from build123d import *

# Parameters (mm, degrees)
F1_DEPTH = 60
F2_W     = 3
F2_H     = 3
F3_DEPTH = 60
F4_DEPTH = 42
F5_DEPTH = 35
F6_DEPTH = 7


with BuildPart() as f1:
    # F0 (on Front) → F1 (new body)
    with BuildSketch(Plane.XZ):
        with BuildLine():
            Line((-6, 0), (0, 0))
            Line((0, 0), (0, 3))
            Line((0, 3), (-6.3828637444, 3.5))
            ThreePointArc((-6.3828637444, 3.5), (-7.5200895217, 3.1043228005), (-8, 2))
            ThreePointArc((-8, 2), (-7.4142135624, 0.5857864376), (-6, 0))
        make_face()
    extrude(amount=F1_DEPTH)

    # F2 (on face) → F3 (join)
    with BuildSketch(Plane.XZ.offset(60)):
        with Locations((1.5, 1.5)):
            Rectangle(F2_W, F2_H)
    extrude(amount=-F3_DEPTH)

    # F4 (cut): a face of the model
    f4_faces = [f1.faces().sort_by_distance(p)[0] for p in [
        (-2.4940313384, -60, 1.6228930979),
    ]]
    extrude(f4_faces, amount=-F4_DEPTH, mode=Mode.SUBTRACT)

    # F5 (add): a face of the model
    f5_faces = [f1.faces().sort_by_distance(p)[0] for p in [
        (-2.4940313384, -18, 1.6228930979),
    ]]
    extrude(f5_faces, amount=F5_DEPTH)

    # F6 (add): a face of the model
    f6_faces = [f1.faces().sort_by_distance(p)[0] for p in [
        (-2.4940313384, -53, 1.6228930979),
    ]]
    extrude(f6_faces, amount=F6_DEPTH)


solid = f1.part
For this review, take the finished solid that the model builds, in its own axes (mm). A direction names the side the tool comes from. Round coordinates to 2 decimals unless told otherwise and drop trailing zeros. Write each loop counter-clockwise with the first axis right and the second up, starting at its lowest first coordinate (ties: lowest second). Pieces come first, ordered by that corner, then holes. Notation, with made-up numbers: (72.25, 28.25) -> (123.25, 28.25) arc R13 cw to (123.25, 50.25) -> close; hole circle Ø1 at (75, 54). An arc over 180 degrees is marked (long way). Put each result on its own line as item: value.
Q1. To check wall thickness, follow L1, parallel to Z at x = 1.5, y = -7; L2, parallel to X at y = -21.5, z = 2.2; L3, parallel to Z at x = -7.25, y = -43. State the ranges of each line that lie inside material, in increasing order. Write a range as [from, to].
Determined:
L1: z = [0, 3]
L2: x = [-7.99, 3]
L3: z = [0.44, 3.3]
Q2. Consider section C-C on z = 0.75. State the section outline as (x, y) points, and give its area (3 significant figures).
Determined:
outline: (-7.56, -60) -> (3, -60) -> (3, 0) -> (-7.56, 0) -> close
area: 634 mm^2
Q3. Consider section A-A on y = -34. State the section outline as (x, z) points, and give its area (3 significant figures).
Determined:
outline: (-8, 2) arc R2 ccw to (-6, 0) -> (3, 0) -> (3, 3) -> (0, 3) -> (-6.38, 3.5) arc R1.5 ccw to start
area: 34.1 mm^2
Q4. Machinability: for faces 1 (the flat face through (1, -30, 3)), 2 (the cylindrical face through (-7.43, -29.58, 0.6)), which of the approach directions +Z, -Z, +X, -X, +Y, -Y give a long, thin tool a straight path to every point of the face, cutting with its end or side? Answer none if there is none.
Determined:
face 1: +Z, +X, +Y, -Y
face 2: -Z, -X, +Y, -Y
Q5. Consider section B-B on x = 0.5. State the section outline as (y, z) points.
Determined:
outline: (-60, 0) -> (0, 0) -> (0, 3) -> (-60, 3) -> close
Q6. Clearance check with flat-ended pins moving along their axes: pin 1 Ø1 at (x, y) = (-5, -47) entering from +Z; pin 2 Ø0.9 at (x, y) = (2, -18.5) entering from +Z. State where each tip first meets the part, or that it passes through.
Determined:
pin 1: stops at z = 3.43
pin 2: stops at z = 3
